Solid Edge part; units mm, degrees
sketch "Sketch1" plane through (0, 0, 0) normal (0, -1, 0) x (1, 0, 0)
  line L0 (-5, 25) -> (-5, 19)
  line L1 (5, 19) -> (-5, 19)
  line L2 (5, 35) -> (5, 19)
  line L3 (5, 35) -> (-90, 35)
  line L4 (-90, 35) -> (-100, 25)
  line L5 (-100, 25) -> (-100, 10)
  line L6 (-100, 10) -> (-90, 10)
  line L7 (-90, 10) -> (-90, 20.8579)
  line L8 (-90, 20.8579) -> (-85.8579, 25)
  line L9 (-85.8579, 25) -> (-45, 25)
  line L10 (-45, 25) -> (-45, 5)
  arc A0 (-35, 5) -> (-45, 5) centre (-40, 5) cw
  line L11 (-35, 5) -> (-35, 25)
  line L12 (-35, 25) -> (-5, 25)
  dimension "D1" = 35
extrude "Protrusion1" add sketch "Sketch1" along normal mid plane 10
fillet "Round_1" radius 5 4 edges at (-5, -5, 22) (-5, 5, 22) (5, 5, 27) (5, -5, 27)
sketch "Sketch2" plane through (0, 0, 0) normal (0, -1, 0) x (1, 0, 0)
  circle A0 centre (-80, 30) radius 1.35
extrude "ExtrudedCutout_3" cut sketch "Sketch2" along normal mid plane 29.2691
sketch "Sketch3" plane through (-100, 0, 15) normal (-1, 0, 0) x (0, 0, -1)
  line L0 (5, 2.5) -> (-3, 2.5)
  line L1 (-3, 2.5) -> (-3, -2.5)
  line L2 (-3, -2.5) -> (5, -2.5)
  line L3 (5, -2.5) -> (5, 2.5)
  dimension "D1" = 5
  dimension "D2" = 3
extrude "Cutout1" cut sketch "Sketch3" against normal blind 5
fillet "Round_6" radius 2 1 edges at (-100, 2.5, 14)
hole "Hole_1" at (-40, -5, 5) direction (0, 1, 0) diameter 4.2 end up to next
fillet "Round_7" radius 5 2 edges at (-45, 0, 25) (-35, 0, 25)
chamfer "Chamfer_4" distance 3.4 angle 60 1 edges at (-5, 0, 19) measured on face at (3.4333, -3.2333, 19)
sketch "Sketch4" plane through (0, 0, 0) normal (0, -1, 0) x (1, 0, 0)
  line L0 (-90, 10) -> (-100, 11.5838)
  line L1 (-100, 11.5838) -> (-100, 10)
  line L2 (-100, 10) -> (-90, 10)
extrude "ExtrudedCutout_5" cut sketch "Sketch4" along normal mid plane 99.8036
properties material "PVC"
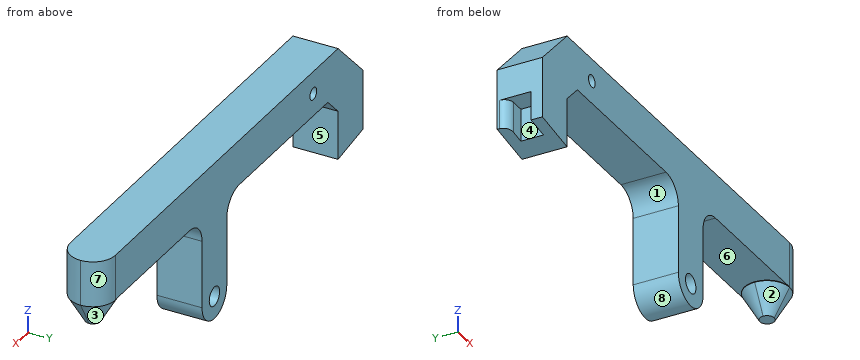
Build history of the part. All positions in model axes, mm. Face numbers are marked on the shaded views. A direction names the side the tool comes from. Round coordinates to 2 decimals unless told otherwise and drop trailing zeros. Write each loop counter-clockwise with the first axis right and the second up, starting at its lowest first coordinate (ties: lowest second). Pieces come first, ordered by that corner, then holes. Notation, with made-up numbers: M 37.25,68.25 L 85.25,68.25 A17 cw 85.25,101.25 Z; hole C 9.25,5.25 d8. An arc over 180 degrees is marked long. Answer as a JSON object with one key per item and string values. Group by question number.
(1) Cut at D-D (y = -3.5). Give the number of separate pieces and of enclosed holes in the cut face, and give its area (3 significant figures).
(2) Which spindle directions (+Z, -Z, +X, -X, +Y, -Y) get a long thin tool onto all of the face, cutting with end or side? Do the marked faces 1, 2, 3 and 4. Say none if no direction does.
(3) Mould opens along X. For the marked faces 5, 6, 7 and 8 say: pulls with the +X half, pulls with the -X half, needs draft (parallel to the pull), parting line crosses it, or undercut.
(4) Flat gauge pins, fed straight in: pin 1 (1 mm diameter, centred on y = 2, z = 26, fed in from -X); pin 2 (3 mm diameter, centred on y = -1.5, z = 9, fed in from +X); pin 3 (1 mm diameter, centred on x = -60.5, z = 23.5, fed in from +Y); pin 4 (1 mm diameter, centred on x = 0, y = -0.5, fed in from -Z). Where does each tip first touch, or does it go through?
(5) Cut at A-A (x = -40). Give the cut face in (y, z), and give its area (3 significant figures).
(6) Drill centre lines: L1, parallel to X at y = 0.5, z = 17; L2, parallel to X at y = 0.75, z = 5; L3, parallel to X at y = -1.5, z = 23. Where is each one in solid material? Low to high.
(7) Cut at C-C (x = -80). Give the cut face in (y, z), and give its area (3 significant figures).
Responses:
{
 "1": {"separate pieces": "1", "enclosed holes": "2", "area": "1,380 mm2"},
 "2": {"face 1": "-Z, +Y, -Y", "face 2": "-Z, -Y", "face 3": "-Z, +X, +Y", "face 4": "-Z, -X"},
 "3": {"face 5": "undercut", "face 6": "undercut", "face 7": "pulls with the +X half", "face 8": "parting line crosses it"},
 "4": {"pin 1": "stops at x = -99.5", "pin 2": "stops at x = -35", "pin 3": "passes through", "pin 4": "stops at z = 19"},
 "5": {"outline": "M -5,0 L 5,0 L 5,2.9 L -5,2.9 Z; M -5,7.1 L 5,7.1 L 5,35 L -5,35 Z", "area": "308 mm2"},
 "6": {"L1": "x = -95 to -90, -45 to -35", "L2": "x = -45 to -42.1, -37.9 to -35", "L3": "x = -100 to -87.86, -46 to -34, -3.61 to 3.61"},
 "7": {"outline": "M -5,25 L 5,25 L 5,28.65 L -5,28.65 Z; M -5,31.35 L 5,31.35 L 5,35 L -5,35 Z", "area": "73.0 mm2"}
}
